Read the model definition and answer for the solid it produces. Units are mm, in the model's axes. Coordinates: 2 decimals unless noted, no trailing zeros. Loops run counter-clockwise (first coordinate to the right, second up) from the corner with the lowest first, then second, coordinate; pieces in that order, holes last. Notation, with made-up numbers: (22, 85.25) -> (65, 85.25) arc R8 cw to (65, 93.25) -> close; hole circle Ø11 at (13.25, 87.5). An arc over 180 degrees is marked (long way). Answer as a JSON object with one key per item and string values. Group by question number.
Q1. The part is cut by section A-A on z = 29. Write down the section's boundary in (x, y), and give its area (3 significant figures).
Q2. The part is cut by section B-B on y = -136. Write down the section's boundary in (x, z).
Q3. The part is cut by section C-C on y = -20. Write down the section's boundary in (x, z), and give its area (3 significant figures).
Q4. Each of these flat-tipped pins is pushed along its axis until it touches: P1, Ø11, axis at y = 41, z = 29.5, coming from the -X side; P2, Ø8, axis at x = -7.5, y = -6.5, coming from the +Z side; P3, Ø12, axis at y = -128, z = 4.5, coming from the -X side. Where does it stop, or does it pass through?
Q5. Straight lines are drawn through the part: line 1 along X through (y, z) = (-197, 16); line 2 along Z through (x, y) = (63, 27.5); line 3 along X through (y, z) = (-90.5, 37.5). For each, find the intervals that lie inside material, in ascending order. Write a range as [from, to].
from build123d import *

# Parameters (mm, degrees)
BOSS_EXTRUDE1_DEPTH = 20
SKETCH2_R           = 5
BOSS_EXTRUDE2_DEPTH = 20
SKETCH3_W           = 200
SKETCH3_H           = 20
BOSS_EXTRUDE3_DEPTH = 50
SKETCH4_W           = 30
SKETCH4_H           = 10
BOSS_EXTRUDE4_DEPTH = 20
SKETCH5_W           = 18
SKETCH5_H           = 10
CUT_EXTRUDE1_DEPTH  = 145.75
SKETCH6_W           = 50
SKETCH6_H           = 20
BOSS_EXTRUDE5_DEPTH = 120
FILLET1_R           = 30
FILLET2_R           = 30
FILLET3_R           = 3
FILLET4_R           = 1


with BuildPart() as part:
    # Sketch1 → Boss-Extrude1 (new body)
    with BuildSketch(Plane.XY):
        Polygon((-100, 0), (-50, 50), (50, 50), (100, 0), (100, -50), (-100, -50), align=None)
    extrude(amount=BOSS_EXTRUDE1_DEPTH)

    # Sketch2 → Boss-Extrude2 (add)
    with BuildSketch(Plane.XY.offset(20)):
        with Locations((-84.27, -20)):
            Circle(SKETCH2_R)
        with Locations((84.27, -20)):
            Circle(SKETCH2_R)
    extrude(amount=BOSS_EXTRUDE2_DEPTH)

    # Sketch3 → Boss-Extrude3 (add)
    with BuildSketch(Plane.XZ.offset(50)):
        with Locations((0, 10)):
            Rectangle(SKETCH3_W, SKETCH3_H)
    extrude(amount=BOSS_EXTRUDE3_DEPTH)

    # Sketch4 → Boss-Extrude4 (add)
    with BuildSketch(Plane.XY.offset(20)):
        with Locations((0, -89.75)):
            Rectangle(SKETCH4_W, SKETCH4_H)
        with Locations((0, 40.86768586)):
            Rectangle(SKETCH4_W, SKETCH4_H)
    extrude(amount=BOSS_EXTRUDE4_DEPTH)

    # Sketch5 → Cut-Extrude1 (cut, through all)
    with BuildSketch(Plane.XZ.offset(94.75)):
        with Locations((0, 29)):
            Rectangle(SKETCH5_W, SKETCH5_H)
    extrude(amount=-CUT_EXTRUDE1_DEPTH, mode=Mode.SUBTRACT)

    # Sketch6 → Boss-Extrude5 (add)
    with BuildSketch(Plane.XZ.offset(100)):
        with Locations((-25, 10)):
            Rectangle(SKETCH6_W, SKETCH6_H)
        with Locations((25, 10)):
            Rectangle(SKETCH6_W, SKETCH6_H)
    extrude(amount=BOSS_EXTRUDE5_DEPTH)

    # Fillet1
    fillet1_edges = [part.edges().sort_by_distance(p)[0] for p in [
        (-100, -100, 10),
        (100, -100, 10),
    ]]
    fillet(fillet1_edges, radius=FILLET1_R)

    # Fillet2
    fillet2_edges = [part.edges().sort_by_distance(p)[0] for p in [
        (-50, -100, 10),
        (50, -100, 10),
    ]]
    fillet(fillet2_edges, radius=FILLET2_R)

    # Fillet3
    fillet3_edges = [part.edges().sort_by_distance(p)[0] for p in [
        (-50, -174.580398915, 20),
        (-50, -174.580398915, 0),
        (50, -174.580398915, 0),
        (50, -174.580398915, 20),
        (0, -220, 0),
        (0, -220, 20),
        (100, -35, 0),
        (92.912878475, -89.364916731, 0),
        (100, -35, 20),
        (-92.912878475, -89.364916731, 20),
        (0, 50, 20),
        (-92.912878475, -89.364916731, 0),
        (92.912878475, -89.364916731, 20),
        (-57.087121525, -109.7958811, 20),
        (-57.087121525, -109.7958811, 0),
        (57.087121525, -109.7958811, 0),
        (57.087121525, -109.7958811, 20),
        (-75, 25, 20),
        (-100, -35, 20),
        (15, -89.75, 40),
        (-15, -89.75, 40),
        (-15, 40.86768586, 40),
        (15, 40.86768586, 40),
        (-100, -35, 0),
        (-75, 25, 0),
        (0, 50, 0),
        (75, 25, 0),
    ]]
    fillet(fillet3_edges, radius=FILLET3_R)

    # Fillet4
    fillet4_edges = [part.edges().sort_by_distance(p)[0] for p in [
        (-89.27, -20, 20),
        (79.27, -20, 20),
    ]]
    fillet(fillet4_edges, radius=FILLET4_R)


solid = part.part
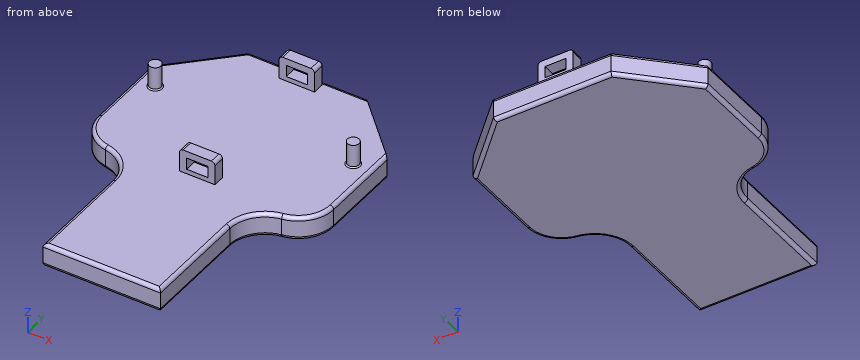
Final values:
{
 "1": {"outline": "circle Ø10 at (-84.27, -20); (-15, -94.75) -> (-9, -94.75) -> (-9, -84.75) -> (-15, -84.75) -> close; (-15, 35.87) -> (-9, 35.87) -> (-9, 45.87) -> (-15, 45.87) -> close; (9, -94.75) -> (15, -94.75) -> (15, -84.75) -> (9, -84.75) -> close; (9, 35.87) -> (15, 35.87) -> (15, 45.87) -> (9, 45.87) -> close; circle Ø10 at (84.27, -20)", "area": "397 mm2"},
 "2": {"outline": "(-50, 3) arc R3 ccw to (-47, 0) -> (47, 0) arc R3 ccw to (50, 3) -> (50, 17) arc R3 ccw to (47, 20) -> (-47, 20) arc R3 ccw to (-50, 17) -> close"},
 "3": {"outline": "(-100, 3) arc R3 ccw to (-97, 0) -> (97, 0) arc R3 ccw to (100, 3) -> (100, 17) arc R3 ccw to (97, 20) -> (90.27, 20) arc R1 cw to (89.27, 21) -> (89.27, 40) -> (79.27, 40) -> (79.27, 21) arc R1 cw to (78.27, 20) -> (-78.27, 20) arc R1 cw to (-79.27, 21) -> (-79.27, 40) -> (-89.27, 40) -> (-89.27, 21) arc R1 cw to (-90.27, 20) -> (-97, 20) arc R3 ccw to (-100, 17) -> close", "area": "4,390 mm2"},
 "4": {"P1": "stops at x = -15", "P2": "stops at z = 20", "P3": "stops at x = -50.87"},
 "5": {"line 1": "x = [-50, 50]", "line 2": "z = [0, 20]", "line 3": "x = [-14.96, 14.96]"}
}
